Design review of the part built by this model. Coordinates are the model's own, in mm. A direction names the side the tool comes from. Coordinates: 2 decimals unless noted, no trailing zeros. Loops run counter-clockwise (first coordinate to the right, second up) from the corner with the lowest first, then second, coordinate; pieces in that order, holes last. Notation, with made-up numbers: M -32,-18.5 L 19,-18.5 A14 ccw 19,-6.5 Z; hole C -28.5,11 d2. An arc over 180 degrees is marked long. Write item = value, one per line. Start each with the question number.
```python
from build123d import *

# Parameters (mm, degrees)
SKETCH1_R           = 8.255
BOSS_EXTRUDE1_DEPTH = 23.495
SKETCH9_R           = 1.905
BOSS_EXTRUDE6_DEPTH = 17.78


with BuildPart() as part:
    # Sketch1 → Boss-Extrude1 (new body)
    with BuildSketch(Plane(origin=(0, 0, 0), x_dir=(1, 0, 0), z_dir=(0, 1, 0))):
        Circle(SKETCH1_R)
    extrude(amount=BOSS_EXTRUDE1_DEPTH)

    # Sketch9 → Boss-Extrude6 (add)
    with BuildSketch(Plane(origin=(0, 23.495, 0), x_dir=(1, 0, 0), z_dir=(0, 1, 0))):
        Polygon((0, 6.892407514), (-5.969, 3.446203757), (-5.969, -3.446203757), (0, -6.892407514), (5.969, -3.446203757), (5.969, 3.446203757), align=None)
        Circle(SKETCH9_R, mode=Mode.SUBTRACT)
    extrude(amount=BOSS_EXTRUDE6_DEPTH)


solid = part.part
```
(1) Take a section at A-A (y = 31.5). State the section outline as (x, z) points (3 decimals), plus the area to 3 significant figures.
(2) Take a section at D-D (y = 20). State the section outline as (x, z) points (3 decimals).
(3) Tool access review of faces 1 (the flat face through (-5.969, 32, 0)), 2 (the flat face through (3.026, 32.261, -5.145)), 3 (the flat face through (-2, 23.495, -6)), 4 (the flat face through (-3.026, 32.261, 5.145)), 5 (the flat face through (2.943, 32.261, 5.193)): name each direction out of +Z, -Z, +X, -X, +Y, -Y from which nothing blocks a thin tool from reaching the whole face with its end or side.
(4) To check wall thickness, follow L1, parallel to X at y = 35.25, z = 0 (3 decimals); L2, parallel to Z at x = 0, y = 29.75 (3 decimals); L3, parallel to Y at x = 6, z = 3.75 (3 decimals). State the ranges of each line that lie inside material, in increasing order.
(5) Take a section at B-B (z = 0). State the section outline as (x, y) points (3 decimals), plus the area to 3 significant figures.
(6) Take a section at C-C (x = 1). State the section outline as (y, z) points (3 decimals).
(7) Insertion check: pin 1 (5 mm diameter, centred on x = -1.5, y = 26.5, fed in from +Z); pin 2 (2.5 mm diameter, centred on x = 0, z = 0, fed in from +Y) (3 decimals); pin 3 (2 mm diameter, centred on y = 28.5, z = -0.5, fed in from -X). Each pin has a flat end and moves straight along its axis. Give the tip position at first contact, or say it passes through.
(8) Mouldability with a two-part tool opening along X and no side actions: class faces 6 (the flat face through (0, 23.495, 0)), 7 (the flat face through (5.969, 32, 0)), 8 (the flat face through (-2.943, 32.261, -5.193)) as +X half, -X half, draft (parallel to the pull), parting line (faces both ways), or undercut.
Results list:
q1.outline = M -5.969,-3.446 L 0,-6.892 L 5.969,-3.446 L 5.969,3.446 L 0,6.892 L -5.969,3.446 Z; hole C 0,0 d3.81
q1.area = 112 mm^2
q2.outline = C 0,0 d16.51
q3.face_1 = +Z, -Z, -X, +Y
q3.face_2 = -Z, +X, +Y
q3.face_3 = +Y
q3.face_4 = +Z, -X, +Y
q3.face_5 = +Z, +X, +Y
q4.L1 = -5.969 to -1.905, 1.905 to 5.969
q4.L2 = -6.892 to -1.905, 1.905 to 6.892
q4.L3 = 0 to 23.495
q5.outline = M -8.255,0 L 8.255,0 L 8.255,23.495 L 5.969,23.495 L 5.969,41.275 L 1.905,41.275 L 1.905,23.495 L -1.905,23.495 L -1.905,41.275 L -5.969,41.275 L -5.969,23.495 L -8.255,23.495 Z
q5.area = 532 mm^2
q6.outline = M 0,-8.194 L 23.495,-8.194 L 23.495,-6.315 L 41.275,-6.315 L 41.275,-1.621 L 23.495,-1.621 L 23.495,1.621 L 41.275,1.621 L 41.275,6.315 L 23.495,6.315 L 23.495,8.194 L 0,8.194 Z
q7.pin_1 = 6.89
q7.pin_2 = 23.495
q7.pin_3 = -5.97
q8.face_6 = undercut
q8.face_7 = +X half
q8.face_8 = -X half
